```python
from build123d import *

# Parameters (mm, degrees)
SKETCH1_R                  = 1.98
SKETCH1_R_2                = 3
SKETCH1_R_3                = 1.75
BASE_FLANGE1_DEPTH         = 3.2
CUT_EXTRUDE1_DEPTH         = 369.458014569
SKETCHED_START             = 74.836838233
SKETCHED_BEND1_DEPTH       = 52.633161767
SKETCHED_START_2           = 87.47
SKETCHED_BEND1_2_DEPTH     = 40
SKETCHED_START_3           = 83.64
SKETCHED_BEND1_3_DEPTH     = 3.2
SKETCH9_R                  = 2.5
CUT_EXTRUDE2_DEPTH         = 379.450932148
FILLET1_R                  = 6
SKETCH10_W                 = 60
SKETCH10_H                 = 50.166277303
CUT_EXTRUDE3_DEPTH         = 379.450932148
FILLET2_R                  = 10
SKETCHED_START_4           = 21.74
SKETCHED_BEND2_DEPTH       = 20
SKETCHED_BEND2_2_DEPTH     = 20
FILLET3_R                  = 5
SKETCH13_R                 = 3
CUT_EXTRUDE4_DEPTH         = 359.024009312
SKETCHED_START_5           = -53.74
SKETCHED_BEND3_DEPTH       = 120
SKETCHED_BEND3_2_DEPTH     = 120
FILLET4_R                  = 20
SKETCHED_START_6           = 175.97
SKETCHED_BEND5_DEPTH       = 66.7
SKETCHED_START_7           = 208.025657316
SKETCHED_BEND5_2_DEPTH     = 27.944342684
SKETCHED_START_8           = 235.97
SKETCHED_BEND5_3_OUTLINE_W = 3.2
SKETCHED_BEND5_3_OUTLINE_H = 20
SKETCHED_BEND5_3_DEPTH     = 6.7
SKETCHED_BEND5_4_DEPTH     = 32.055657316
SKETCHED_START_9           = 70.161438651
SKETCHED_BEND5_5_DEPTH     = 3.2
SKETCHED_BEND5_6_DEPTH     = 3.2
FILLET5_R                  = 4
FILLET6_R                  = 4
FILLET7_R                  = 4


with BuildPart() as part:
    # Base-Flange1: sheet metal written as solids
    # Sketch1 → Base-Flange1 (new body)
    with BuildSketch(Plane(origin=(0, 0, 0), x_dir=(1, 0, 0), z_dir=(0, 1, 0))):
        with BuildLine():
            Line((-86.74, 77.47), (-86.74, -77.47))
            ThreePointArc((-86.74, -77.47), (-83.811067812, -84.541067812), (-76.74, -87.47))
            Line((-76.74, -87.47), (-53.74, -87.47))
            Line((-53.74, -87.47), (-53.74, -325.97))
            Line((-53.74, -325.97), (66.26, -325.97))
            Line((66.26, -325.97), (66.26, -235.97))
            Line((66.26, -235.97), (98.26, -235.97))
            Line((98.26, -235.97), (98.26, -242.67))
            Line((98.26, -242.67), (118.26, -242.67))
            Line((118.26, -242.67), (118.26, -235.97))
            Line((118.26, -235.97), (76.26, -175.97))
            Line((76.26, -175.97), (66.26, -175.97))
            Line((66.26, -175.97), (66.26, -127.47))
            Line((66.26, -127.47), (86.74, -127.47))
            Line((86.74, -127.47), (171.74, -127.47))
            Line((171.74, -127.47), (171.74, -87.47))
            Line((171.74, -87.47), (163.151263871, -74.836838233))
            Line((163.151263871, -74.836838233), (95.540712582, -74.836838233))
            Line((95.540712582, -74.836838233), (89.641340328, -87.47))
            Line((89.641340328, -87.47), (86.74, -87.47))
            Line((86.74, -87.47), (86.74, 77.47))
            ThreePointArc((86.74, 77.47), (83.811067812, 84.541067812), (76.74, 87.47))
            Line((76.74, 87.47), (41.74, 87.47))
            Line((41.74, 87.47), (41.74, 157.47))
            Line((41.74, 157.47), (21.74, 157.47))
            Line((21.74, 157.47), (21.74, 87.47))
            Line((21.74, 87.47), (-76.74, 87.47))
            ThreePointArc((-76.74, 87.47), (-83.811067812, 84.541067812), (-86.74, 77.47))
        make_face()
        with Locations(Location((-78.74, 77.47, 0), (0, 0, 270))):
            Circle(SKETCH1_R, mode=Mode.SUBTRACT)
        with Locations(Location((-78.74, -77.47, 0), (0, 0, 270))):
            Circle(SKETCH1_R, mode=Mode.SUBTRACT)
        with Locations(Location((78.74, -77.47, 0), (0, 0, 270))):
            Circle(SKETCH1_R, mode=Mode.SUBTRACT)
        with Locations(Location((78.74, 54.61, 0), (0, 0, 270))):
            Circle(SKETCH1_R, mode=Mode.SUBTRACT)
        with Locations(Location((61.74, 81.47, 0), (0, 0, 270))):
            Circle(SKETCH1_R_2, mode=Mode.SUBTRACT)
        with Locations(Location((66.74, 50.47, 0), (0, 0, 270))):
            Circle(SKETCH1_R_3, mode=Mode.SUBTRACT)
        with Locations(Location((66.74, -52.53, 0), (0, 0, 270))):
            Circle(SKETCH1_R_3, mode=Mode.SUBTRACT)
    extrude(amount=BASE_FLANGE1_DEPTH)

    # Sketch6 → Cut-Extrude1 (cut, through all)
    with BuildSketch(Plane(origin=(0, 3.2, 0), x_dir=(1, 0, 0), z_dir=(0, 1, 0))):
        Polygon((86.74, -68.47), (82.74, -72.47), (82.74, -87.47), (86.74, -87.47), align=None)
    extrude(amount=-CUT_EXTRUDE1_DEPTH, mode=Mode.SUBTRACT)

    # Sketched Bend1: read off the stored shape, not the designer's step
    # Sketched Bend1 outline → Sketched Bend1 (cut)
    with BuildSketch(Plane.XY.offset(SKETCHED_START)):
        with BuildLine():
            Line((171.74, 3.2), (86.770471243, 3.2))
            ThreePointArc((86.770471243, 3.2), (85.413093209, 0.903736739), (82.9034, 0))
            Line((82.9034, 0), (171.74, 0))
            Line((171.74, 0), (171.74, 3.2))
        make_face()
    extrude(amount=SKETCHED_BEND1_DEPTH, mode=Mode.SUBTRACT)

    # Sketched Bend1 2 outline → Sketched Bend1 2 (add)
    with BuildSketch(Plane.XY.offset(SKETCHED_START_2)):
        with BuildLine():
            Line((86.84, 89.102877303), (83.64, 89.102877303))
            Line((83.64, 89.102877303), (83.64, 3.9366))
            ThreePointArc((83.64, 3.9366), (83.424254855, 3.415745145), (82.9034, 3.2))
            Line((82.9034, 3.2), (86.770471243, 3.2))
            ThreePointArc((86.770471243, 3.2), (86.822579265, 3.566662908), (86.84, 3.9366))
            Line((86.84, 3.9366), (86.84, 89.102877303))
        make_face()
    extrude(amount=SKETCHED_BEND1_2_DEPTH)

    # Sketched Bend1 3 outline → Sketched Bend1 3 (add)
    with BuildSketch(Plane.YZ.offset(SKETCHED_START_3)):
        Polygon((12.903589884, 74.836838233), (80.514141174, 74.836838233), (89.102877303, 87.47), (7.004217631, 87.47), align=None)
    extrude(amount=SKETCHED_BEND1_3_DEPTH)

    # Sketch9 → Cut-Extrude2 (cut, through all)
    with BuildSketch(Plane.ZY.offset(-83.64)):
        with Locations(Location((93.47, 83.102877303, 0), (0, 0, 270))):
            Circle(SKETCH9_R)
        with Locations(Location((117.47, 10.102877303, 0), (0, 0, 270))):
            Circle(SKETCH9_R)
    extrude(amount=-CUT_EXTRUDE2_DEPTH, mode=Mode.SUBTRACT)

    # Fillet1
    fillet1_edges = [part.edges().sort_by_distance(p)[0] for p in [
        (85.24, 7.004217631, 87.47),
        (85.24, 12.903589884, 74.836838233),
        (85.24, 80.514141174, 74.836838233),
        (85.24, 89.102877303, 87.47),
        (85.24, 89.102877303, 127.47),
    ]]
    fillet(fillet1_edges, radius=FILLET1_R)

    # Sketch10 → Cut-Extrude3 (cut, through all)
    with BuildSketch(Plane.ZY.offset(-83.64)):
        with Locations((120.47, 44.019738651)):
            Rectangle(SKETCH10_W, SKETCH10_H)
    extrude(amount=-CUT_EXTRUDE3_DEPTH, mode=Mode.SUBTRACT)

    # Fillet2
    fillet2_edges = [part.edges().sort_by_distance(p)[0] for p in [
        (85.24, 18.9366, 90.47),
        (85.24, 69.102877303, 127.47),
        (85.24, 69.102877303, 90.47),
    ]]
    fillet(fillet2_edges, radius=FILLET2_R)

    # Sketched Bend2: read off the stored shape, not the designer's step
    # Sketched Bend2 outline → Sketched Bend2 (cut)
    with BuildSketch(Plane.YZ.offset(SKETCHED_START_4)):
        with BuildLine():
            Line((3.2, -157.47), (3.2, -117.400471243))
            ThreePointArc((3.2, -117.400471243), (0.903736739, -116.043093209), (0, -113.5334))
            Line((0, -113.5334), (0, -157.47))
            Line((0, -157.47), (3.2, -157.47))
        make_face()
    extrude(amount=SKETCHED_BEND2_DEPTH, mode=Mode.SUBTRACT)

    # Sketched Bend2 2 outline → Sketched Bend2 2 (add)
    with BuildSketch(Plane.YZ.offset(SKETCHED_START_4)):
        with BuildLine():
            Line((44.202877303, -114.27), (3.9366, -114.27))
            ThreePointArc((3.9366, -114.27), (3.415745145, -114.054254855), (3.2, -113.5334))
            Line((3.2, -113.5334), (3.2, -117.400471243))
            ThreePointArc((3.2, -117.400471243), (3.566662908, -117.452579265), (3.9366, -117.47))
            Line((3.9366, -117.47), (44.202877303, -117.47))
            Line((44.202877303, -117.47), (44.202877303, -114.27))
        make_face()
    extrude(amount=SKETCHED_BEND2_2_DEPTH)

    # Fillet3
    fillet3_edges = [part.edges().sort_by_distance(p)[0] for p in [
        (85.24, 18.9366, 127.47),
    ]]
    fillet(fillet3_edges, radius=FILLET3_R)

    # Sketch13 → Cut-Extrude4 (cut, through all)
    with BuildSketch(Plane.XZ):
        with Locations(Location((31.74, -107.13, 0), (0, 0, 270))):
            Circle(SKETCH13_R)
    extrude(amount=-CUT_EXTRUDE4_DEPTH, mode=Mode.SUBTRACT)

    # Sketched Bend3: read off the stored shape, not the designer's step
    # Sketched Bend3 outline → Sketched Bend3 (cut)
    with BuildSketch(Plane.YZ.offset(SKETCHED_START_5)):
        with BuildLine():
            ThreePointArc((0, 238.7334), (0.903736739, 241.243093209), (3.2, 242.600471243))
            Line((3.2, 242.600471243), (3.2, 325.97))
            Line((3.2, 325.97), (0, 325.97))
            Line((0, 325.97), (0, 238.7334))
        make_face()
    extrude(amount=SKETCHED_BEND3_DEPTH, mode=Mode.SUBTRACT)

    # Sketched Bend3 2 outline → Sketched Bend3 2 (add)
    with BuildSketch(Plane.YZ.offset(SKETCHED_START_5)):
        with BuildLine():
            Line((87.502877303, 242.67), (3.9366, 242.67))
            ThreePointArc((3.9366, 242.67), (3.566662908, 242.652579265), (3.2, 242.600471243))
            Line((3.2, 242.600471243), (3.2, 238.7334))
            ThreePointArc((3.2, 238.7334), (3.415745145, 239.254254855), (3.9366, 239.47))
            Line((3.9366, 239.47), (87.502877303, 239.47))
            Line((87.502877303, 239.47), (87.502877303, 242.67))
        make_face()
    extrude(amount=SKETCHED_BEND3_2_DEPTH)

    # Fillet4
    fillet4_edges = [part.edges().sort_by_distance(p)[0] for p in [
        (-53.74, 87.502877303, 241.07),
        (66.26, 87.502877303, 241.07),
    ]]
    fillet(fillet4_edges, radius=FILLET4_R)

    # Sketched Bend5: read off the stored shape, not the designer's step
    # Sketched Bend5 outline → Sketched Bend5 (cut)
    with BuildSketch(Plane.XY.offset(SKETCHED_START_6)):
        with BuildLine():
            ThreePointArc((69.424838651, 3.2), (71.93453186, 2.296263261), (73.291909894, 0))
            Line((73.291909894, 0), (118.26, 0))
            Line((118.26, 0), (118.26, 3.2))
            Line((118.26, 3.2), (69.424838651, 3.2))
        make_face()
    extrude(amount=SKETCHED_BEND5_DEPTH, mode=Mode.SUBTRACT)

    # Sketched Bend5 2 outline → Sketched Bend5 2 (add)
    with BuildSketch(Plane.XY.offset(SKETCHED_START_7)):
        with BuildLine():
            ThreePointArc((73.361438651, -0.7366), (73.344017916, -0.366662908), (73.291909894, 0))
            Line((73.291909894, 0), (69.424838651, 0))
            ThreePointArc((69.424838651, 0), (69.945693506, -0.215745145), (70.161438651, -0.7366))
            Line((70.161438651, -0.7366), (70.161438651, -25.901438651))
            Line((70.161438651, -25.901438651), (73.361438651, -25.901438651))
            Line((73.361438651, -25.901438651), (73.361438651, -0.7366))
        make_face()
    extrude(amount=SKETCHED_BEND5_2_DEPTH)

    # Sketched Bend5 3 outline → Sketched Bend5 3 (add)
    with BuildSketch(Plane.XY.offset(SKETCHED_START_8)):
        with Locations((71.761438651, -35.901438651)):
            Rectangle(SKETCHED_BEND5_3_OUTLINE_W, SKETCHED_BEND5_3_OUTLINE_H)
    extrude(amount=SKETCHED_BEND5_3_DEPTH)

    # Sketched Bend5 4 outline → Sketched Bend5 4 (add)
    with BuildSketch(Plane.XY.offset(SKETCHED_START_6)):
        with BuildLine():
            ThreePointArc((73.361438651, -0.7366), (73.344017916, -0.366662908), (73.291909894, 0))
            Line((73.291909894, 0), (69.424838651, 0))
            ThreePointArc((69.424838651, 0), (69.945693506, -0.215745145), (70.161438651, -0.7366))
            Line((70.161438651, -0.7366), (70.161438651, -25.901438651))
            Line((70.161438651, -25.901438651), (73.361438651, -25.901438651))
            Line((73.361438651, -25.901438651), (73.361438651, -0.7366))
        make_face()
    extrude(amount=SKETCHED_BEND5_4_DEPTH)

    # Sketched Bend5 5 outline → Sketched Bend5 5 (cut)
    with BuildSketch(Plane.YZ.offset(SKETCHED_START_9)):
        Polygon((-3.901438651, 175.97), (-25.901438651, 207.398571429), (-25.901438651, 175.97), align=None)
    extrude(amount=SKETCHED_BEND5_5_DEPTH, mode=Mode.SUBTRACT)

    # Sketched Bend5 6 outline → Sketched Bend5 6 (add)
    with BuildSketch(Plane.YZ.offset(SKETCHED_START_9)):
        Polygon((-25.901438651, 235.97), (-45.901438651, 235.97), (-25.901438651, 207.398571429), align=None)
    extrude(amount=SKETCHED_BEND5_6_DEPTH)

    # Fillet5
    fillet5_edges = [part.edges().sort_by_distance(p)[0] for p in [
        (41.74, 44.202877303, -115.87),
        (21.74, 44.202877303, -115.87),
    ]]
    fillet(fillet5_edges, radius=FILLET5_R)

    # Fillet6
    fillet6_edges = [part.edges().sort_by_distance(p)[0] for p in [
        (71.761438651, -45.901438651, 235.97),
        (71.761438651, -45.901438651, 242.67),
        (71.761438651, -25.901438651, 242.67),
        (71.761438651, -3.901438651, 175.97),
    ]]
    fillet(fillet6_edges, radius=FILLET6_R)

    # Fillet7
    fillet7_edges = [part.edges().sort_by_distance(p)[0] for p in [
        (71.761438651, -25.901438651, 235.97),
    ]]
    fillet(fillet7_edges, radius=FILLET7_R)


solid = part.part
```
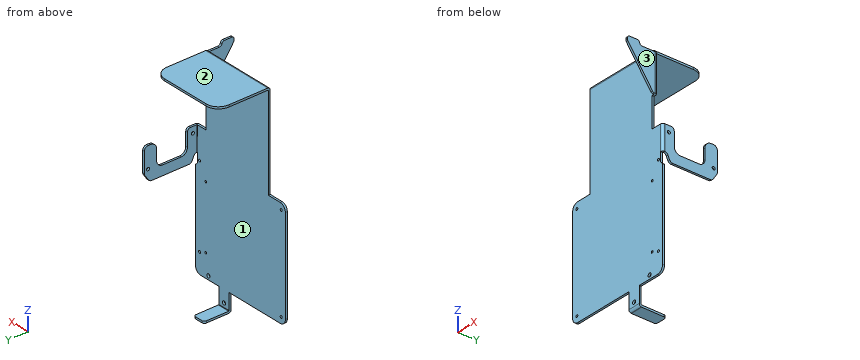
The model under review builds one solid part; all positions refer to its coordinate system, in mm. Face numbers are marked on the shaded views. Round coordinates to 2 decimals unless told otherwise and drop trailing zeros. Loops run counter-clockwise (first coordinate to the right, second up) from the corner with the lowest first, then second, coordinate; pieces in that order, holes last. Notation, with made-up numbers: (56.5, 33) - (94.5, 33) arc R30 cw to (94.5, 65) - close; hole circle Ø1 at (75.5, -32). An arc over 180 degrees is marked (long way). Write each question's results on one line, items separated by ' | '. Start each with the question number.
Q1. Draft analysis for pull direction Z (two halves, no side actions). For the marked faces 1, 2 and 3, state which applies: pulls with the +Z half, pulls with the -Z half, needs draft (parallel to the pull), parting line crosses it, or undercut.
Q2. Take a section at C-C on z = 189. Give the boundary of the cut face in (x, y).
Q3. Take a section at B-B on x = 11. Give the boundary of the cut face in (y, z), plus the area to 3 significant figures.
Q4. Take a section at A-A on y = 55. Give the boundary of the cut face in (x, z), plus the area to 3 significant figures.
Q5. Insertion check: P1, Ø6, axis at y = 10.1, z = 117.47, coming from the +X side; P2, Ø2.5, axis at x = -71, y = 2.5, coming from the +Z side; P3, Ø2.5, axis at x = -1, z = 241, coming from the +Y side; P4, Ø3.5, axis at x = 86, y = 41, coming from the +Z side. Each pin has a flat end and moves straight along its axis. Give the tip position at first contact, or say it passes through.
Q6. Take a section at D-D on y = -17. Give the boundary of the cut face in (x, z).
Q7. Wall thickness on line 1 along X through (y, z) = (0.75, 52.53); line 2 along Y through (x, z) = (-51.5, -32); line 3 along X through (y, z) = (2, -54): over which ranges is each line inside the solid? List them lowest first. Write a range as [from, to].
Data:
1) face 1: undercut | face 2: pulls with the +Z half | face 3: needs draft
2) outline: (-53.74, 0) - (69.42, 0) arc R0.74 cw to (70.16, -0.74) - (70.16, -13.02) - (73.36, -13.02) - (73.36, -0.74) arc R3.94 ccw to (69.42, 3.2) - (-53.74, 3.2) - close
3) outline: (0, -87.47) - (3.2, -87.47) - (3.2, 238.73) arc R0.74 cw to (3.94, 239.47) - (87.5, 239.47) - (87.5, 242.67) - (3.94, 242.67) arc R3.94 ccw to (0, 238.73) - close | area: 1,320 mm²
4) outline: (-53.74, 239.47) - (66.26, 239.47) - (66.26, 242.67) - (-53.74, 242.67) - close; (83.64, 74.84) - (86.84, 74.84) - (86.84, 90.47) - (83.64, 90.47) - close | area: 434 mm²
5) P1: stops at x = 86.84 | P2: stops at z = 87.47 | P3: stops at y = 87.5 | P4: stops at z = 90.47
6) outline: (70.16, 194.68) - (73.36, 194.68) - (73.36, 235.97) - (70.16, 235.97) - close
7) line 1: x = [-86.74, 64.99], [68.49, 86.74] | line 2: y = [0, 3.2] | line 3: x = [-86.74, 76.86], [80.62, 86.74]
